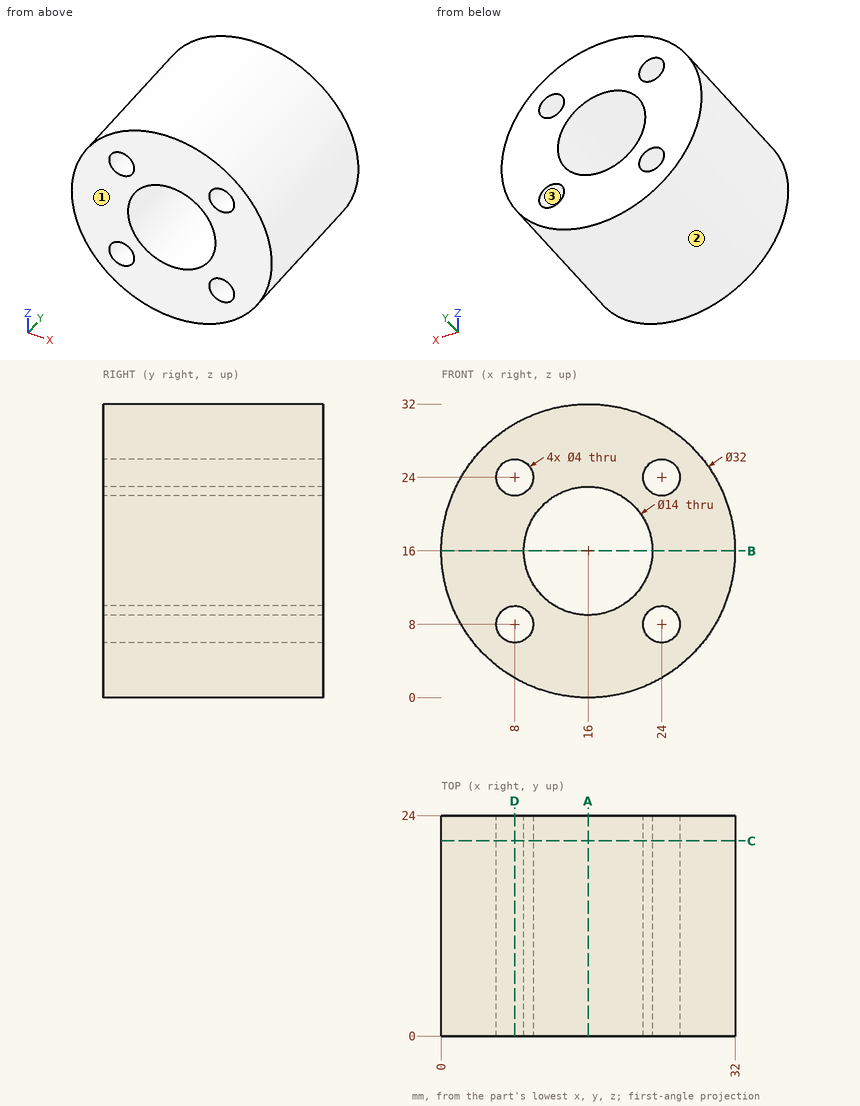
Can you work these out from the drawing? Everything is in mm from the part's minimum corner. Give positions to 0.01 mm unless a question says otherwise; leave off trailing zeros. Loops run counter-clockwise (first coordinate to the right, second up) from the corner with the lowest first, then second, coordinate; pieces in that order, holes last. Notation, with made-up numbers: (20.25, 72) - (31.25, 72) arc R15 ccw to (31.25, 79) - close; hole circle Ø1 at (-22, -12.5). An arc over 180 degrees is marked (long way). Use one line per item in the form item = value.
1. I'm going to push flat-ended pins straight in: pin 1 Ø2.5 at (x, z) = (8, 8) entering from +Y; pin 2 Ø5 at (x, y) = (8, 7.5) entering from +Z (3 decimals); pin 3 Ø2 at (y, z) = (16.5, 19) entering from +X; pin 4 Ø4 at (x, y) = (20, 17) entering from -Z. Where does each tip first touch, or does it pass through?
Response values:
pin_1 = through
pin_2 = 31.025
pin_3 = 31.87
pin_4 = 0.13
2. I want a section at D-D (x = 8). Please give me the cut outline in (y, z), and give its area (3 significant figures).
Response values:
outline = (0, 2.14) - (24, 2.14) - (24, 6) - (0, 6) - close; (0, 10) - (24, 10) - (24, 22) - (0, 22) - close; (0, 26) - (24, 26) - (24, 29.86) - (0, 29.86) - close
area = 473 mm²
3. I want a section at A-A (x = 16). Please give me the cut outline in (y, z), and give its area (3 significant figures).
Response values:
outline = (0, 0) - (24, 0) - (24, 9) - (0, 9) - close; (0, 23) - (24, 23) - (24, 32) - (0, 32) - close
area = 432 mm²
4. I want a section at B-B (z = 16). Please give me the cut outline in (x, y), and give its area (3 significant figures).
Response values:
outline = (0, 0) - (9, 0) - (9, 24) - (0, 24) - close; (23, 0) - (32, 0) - (32, 24) - (23, 24) - close
area = 432 mm²
5. Thinking about a two-plate mould opening in Z: for the marked faces 1, 2 and 3, which applies, released by +Z, released by -Z, zero draft, split by the parting line, or undercut?
Response values:
face_1 = zero draft
face_2 = split by the parting line
face_3 = undercut
6. I want a section at C-C (y = 21.25). Please give me the cut outline in (x, z), and give its area (3 significant figures).
Response values:
outline = circle Ø32 at (16, 16); hole circle Ø4 at (8, 8); hole circle Ø4 at (8, 24); hole circle Ø14 at (16, 16); hole circle Ø4 at (24, 8); hole circle Ø4 at (24, 24)
area = 600 mm²
7. I need wall thicknesses on probe 1 along Z at (x, y) = (24.5, 15); probe 2 along Z at (x, y) = (8, 13.75); probe 3 along X at (y, z) = (14.5, 25.5). Which ranges of each line are inside material? Lowest first, please.
Response values:
probe_1 = 2.44 to 6.06, 9.94 to 22.06, 25.94 to 29.56
probe_2 = 2.14 to 6, 10 to 22, 26 to 29.86
probe_3 = 3.13 to 6.68, 9.32 to 22.68, 25.32 to 28.87
